Geometry check sheet. Reference: the model listing, model coordinates, mm. Give positions to 0.01 mm unless a question says otherwise; leave off trailing zeros. Write each loop counter-clockwise with the first axis right and the second up, starting at its lowest first coordinate (ties: lowest second). Pieces come first, ordered by that corner, then holes. Notation, with made-up numbers: (-10, 55.5) -> (17, 55.5) arc R27 cw to (17, 88.5) -> close; hole circle Ø11 at (88.5, -29.5). An arc over 180 degrees is marked (long way). Write item = value, one per line. Start each with the question number.
1. Cross-section at B-B, the plane z = -13. State how many separate pieces and enclosed holes the cut face has, plus the area to 3 significant figures.
2. Thickness scan on line 1 along X through (y, z) = (-6241, -11.25); line 2 along X through (y, z) = (-6240.5, -3); line 3 along X through (y, z) = (-6272, -13.25). Record the ranges inside material, lowest first.
3. Cross-section at D-D, the plane y = -6330.5. Record the cut outline in (x, z) (3 decimals).
4. Cross-section at C-C, the plane x = 11943.5. Record the cut outline in (y, z).
5. Cross-section at A-A, the plane y = -6233.5. Record the cut outline in (x, z) (3 decimals).
6. Depth check by flat-ended pin: P1, Ø19.5, axis at x = 12248.5, y = -6261, coming from the +Z side (3 decimals); P2, Ø1.5, axis at x = 11723.5, z = -1.5, coming from the +Y side; P3, Ø5, axis at x = 11726.76, y = -6179.5, coming from the +Z side. Enter the tip coordinate at first touch or a pass-through.
```python
from build123d import *

# Parameters (mm, degrees)
EXTRUDE1_DEPTH     = 17.78
SKETCH3_W          = 44.45
SKETCH3_H          = 17.78
CUT_EXTRUDE1_DEPTH = 5.08
SKETCH4_W          = 17.78
SKETCH4_H          = 171.45
CUT_EXTRUDE2_DEPTH = 9.525
CUT_EXTRUDE3_START = -17.78
SKETCH5_R          = 1.5875
SKETCH5_R_2        = 3.302
CUT_EXTRUDE3_DEPTH = 17.78


with BuildPart() as part:
    # Sketch2 → Extrude1 (new body)
    with BuildSketch(Plane.XY):
        Polygon((12254.441666666, -6342.0625), (12254.441666666, -6170.6125), (12209.991666666, -6170.6125), (12209.991666666, -6188.3925), (12127.441666666, -6188.3925), (12127.441666666, -6292.5325), (11822.641666666, -6292.5325), (11822.641666666, -6188.3925), (11740.091666666, -6188.3925), (11740.091666666, -6170.6125), (11695.641666666, -6170.6125), (11695.641666666, -6342.0625), align=None)
    extrude(amount=-EXTRUDE1_DEPTH)

    # Sketch3 → Cut-Extrude1 (cut)
    with BuildSketch(Plane.XY):
        with Locations((11717.866666666, -6179.5025)):
            Rectangle(SKETCH3_W, SKETCH3_H)
        with Locations((12232.216666666, -6179.5025)):
            Rectangle(SKETCH3_W, SKETCH3_H)
    extrude(amount=-CUT_EXTRUDE1_DEPTH, mode=Mode.SUBTRACT)

    # Sketch4 → Cut-Extrude2 (cut)
    with BuildSketch(Plane.XY):
        with Locations((11704.531666666, -6256.3375)):
            Rectangle(SKETCH4_W, SKETCH4_H)
        with Locations((12245.551666666, -6256.3375)):
            Rectangle(SKETCH4_W, SKETCH4_H)
    extrude(amount=-CUT_EXTRUDE2_DEPTH, mode=Mode.SUBTRACT)

    # Sketch5 → Cut-Extrude3 (cut)
    with BuildSketch(Plane.XY.offset(CUT_EXTRUDE3_START)):
        with Locations((11704.531666666, -6314.148958334)):
            Circle(SKETCH5_R)
        with Locations((11704.531666666, -6256.734375)):
            Circle(SKETCH5_R)
        with Locations((11704.531666666, -6199.319791666)):
            Circle(SKETCH5_R)
        with Locations((11726.756666666, -6179.5025)):
            Circle(SKETCH5_R)
        with Locations((11748.981666666, -6208.7125)):
            Circle(SKETCH5_R)
        with Locations((11748.981666666, -6272.2125)):
            Circle(SKETCH5_R)
        with Locations((11790.256666666, -6301.4225)):
            Circle(SKETCH5_R)
        with Locations((11913.446666666, -6301.4225)):
            Circle(SKETCH5_R)
        with Locations((12036.636666666, -6301.4225)):
            Circle(SKETCH5_R)
        with Locations((12159.826666666, -6301.4225)):
            Circle(SKETCH5_R)
        with Locations((12245.551666666, -6314.148958334)):
            Circle(SKETCH5_R)
        with Locations((12245.551666666, -6256.734375)):
            Circle(SKETCH5_R)
        with Locations((12201.101666666, -6272.2125)):
            Circle(SKETCH5_R)
        with Locations((12201.101666666, -6208.7125)):
            Circle(SKETCH5_R)
        with Locations((12245.551666666, -6199.319791666)):
            Circle(SKETCH5_R)
        with Locations((12223.326666666, -6179.5025)):
            Circle(SKETCH5_R)
        with Locations((11742.336730696, -6186.14743597)):
            Circle(SKETCH5_R_2)
        with Locations((12207.746602636, -6186.14743597)):
            Circle(SKETCH5_R_2)
    extrude(amount=CUT_EXTRUDE3_DEPTH, mode=Mode.SUBTRACT)


solid = part.part
```
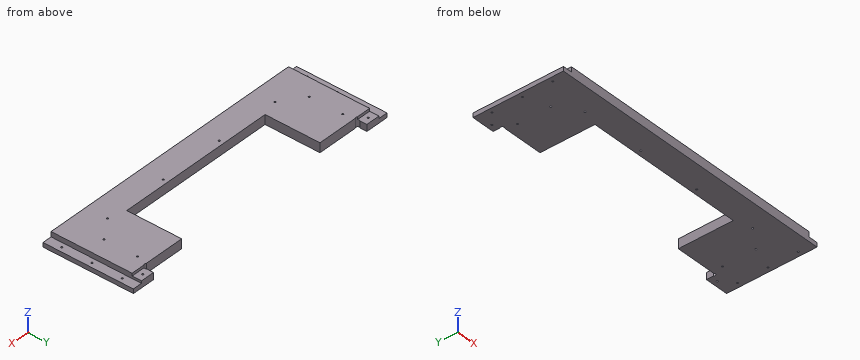
Answers:
q1.separate_pieces = 1
q1.enclosed_holes = 16
q1.area = 55,600 mm^2
q2.line_1 = 11695.64 to 11822.64, 12127.44 to 12254.44
q2.line_2 = 11713.42 to 11822.64, 12127.44 to 12236.66
q2.line_3 = 11695.64 to 11747.41, 11750.55 to 11822.64, 12127.44 to 12199.53, 12202.67 to 12254.44
q3.outline = (11695.642, -17.78) -> (12254.442, -17.78) -> (12254.442, -9.525) -> (12236.662, -9.525) -> (12236.662, 0) -> (11713.422, 0) -> (11713.422, -9.525) -> (11695.642, -9.525) -> close
q4.outline = (-6342.06, -17.78) -> (-6292.53, -17.78) -> (-6292.53, 0) -> (-6342.06, 0) -> close
q5.outline = (11695.642, -17.78) -> (11822.642, -17.78) -> (11822.642, 0) -> (11713.422, 0) -> (11713.422, -9.525) -> (11695.642, -9.525) -> close; (12127.442, -17.78) -> (12254.442, -17.78) -> (12254.442, -9.525) -> (12236.662, -9.525) -> (12236.662, 0) -> (12127.442, 0) -> close
q6.P1 = -9.525
q6.P2 = -6188.39
q6.P3 = -5.08
